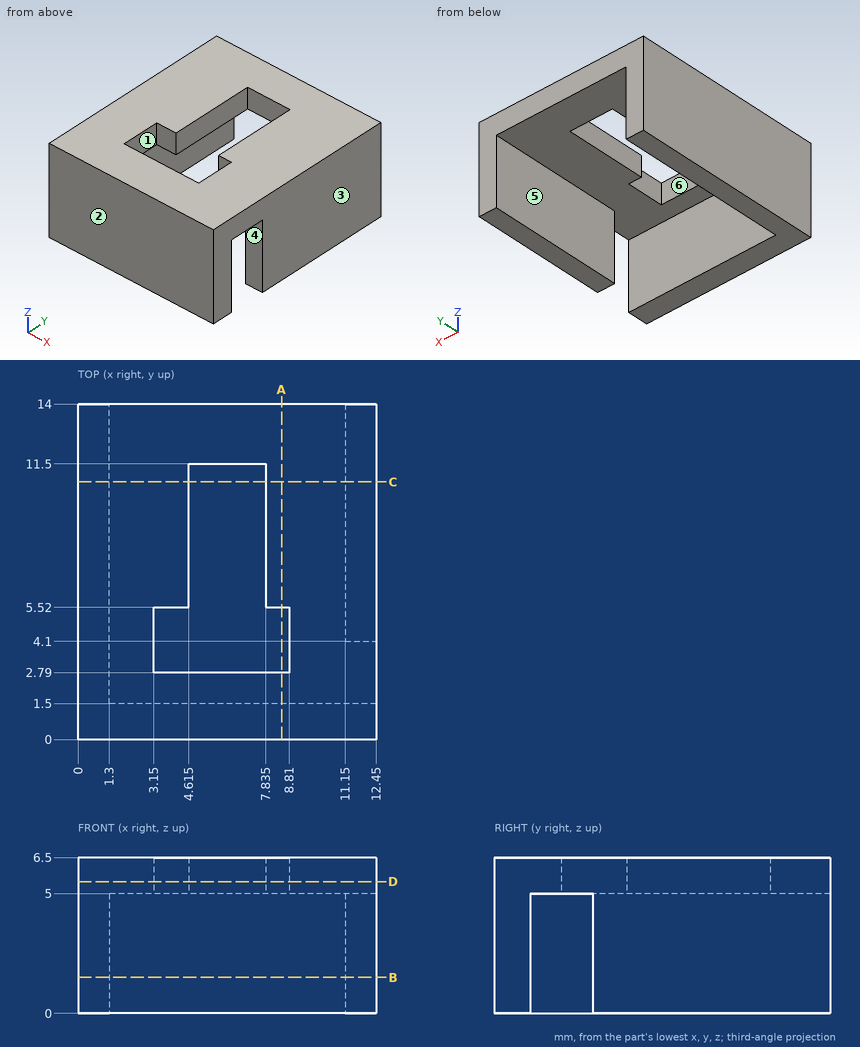
Source: three-view drawing plus pictorial views. Frame: mm from the lowest corner of the part. A direction names the side the tool comes from. Round coordinates to 2 decimals unless told otherwise and drop trailing zeros. Write each loop counter-clockwise with the first axis right and the second up, starting at its lowest first coordinate (ties: lowest second). Pieces come first, ordered by that corner, then holes. Notation, with made-up numbers: M 78,-25.75 L 120,-25.75 A23 cw 120,0.25 Z; hole C 53.5,68.25 d11. An arc over 180 degrees is marked long. Write item = value, one per line.
Item 1: Section query D-D on z = 5.5. Return loops of the section in (x, y) (3 decimals), then the cut area to 3 significant figures.
Findings:
outline = M 0,0 L 12.45,0 L 12.45,14 L 0,14 Z; hole M 3.15,2.79 L 8.81,2.79 L 8.81,5.52 L 7.835,5.52 L 7.835,11.5 L 4.615,11.5 L 4.615,5.52 L 3.15,5.52 Z
area = 140 mm^2
Item 2: Pin query (flat end, axial travel): P1, Ø3.5, axis at x = 4.5, y = 10, coming from the -Z side. Return the tip coordinate at first contact, or that it passes through.
Findings:
P1 = 5
Item 3: Pull-direction query (X, two-part tool) for the marked faces 1, 2 and 3; classes: pulls with the +X half, pulls with the -X half, needs draft (parallel to the pull), parting line crosses it, or undercut.
Findings:
face_1 = undercut
face_2 = needs draft
face_3 = pulls with the +X half
Item 4: Section query A-A on x = 8.5. Return loops of the section in (y, z), then the cut area to 3 significant figures.
Findings:
outline = M 0,0 L 1.5,0 L 1.5,5 L 2.79,5 L 2.79,6.5 L 0,6.5 Z; M 5.52,5 L 14,5 L 14,6.5 L 5.52,6.5 Z
area = 24.4 mm^2
Item 5: Section query C-C on y = 10.75. Return loops of the section in (x, z) (3 decimals), then the cut area to 3 significant figures.
Findings:
outline = M 0,0 L 1.3,0 L 1.3,5 L 4.615,5 L 4.615,6.5 L 0,6.5 Z; M 7.835,5 L 11.15,5 L 11.15,0 L 12.45,0 L 12.45,6.5 L 7.835,6.5 Z
area = 26.8 mm^2
Item 6: Access query for the marked faces 4, 5 and 6. Directions: +Z, -Z, +X, -X, +Y, -Y. A direction counts if a zero-diameter tool reaches every point of the face in a straight line with its end or side. Return the directions, or none.
Findings:
face_4 = -Z, +X
face_5 = -Z, +Y
face_6 = +Z, -Z
Item 7: Material intervals for line 1 along X through (y, z) = (10.75, 2.25); line 2 along X through (y, z) = (3, 5.5); line 3 along Z through (x, y) = (2.75, 4.5), sorted ascending. Write a range as [from, to].
Findings:
line_1 = [0, 1.3], [11.15, 12.45]
line_2 = [0, 3.15], [8.81, 12.45]
line_3 = [5, 6.5]
Item 8: Section query B-B on z = 1.5. Return loops of the section in (x, y).
Findings:
outline = M 0,0 L 12.45,0 L 12.45,1.5 L 1.3,1.5 L 1.3,14 L 0,14 Z; M 11.15,4.1 L 12.45,4.1 L 12.45,14 L 11.15,14 Z
